Build history of the part. All positions in model axes, mm. Face numbers are marked on the shaded views. A direction names the side the tool comes from. Give positions to 0.01 mm unless a question says otherwise; leave off trailing zeros. Write each loop counter-clockwise with the first axis right and the second up, starting at its lowest first coordinate (ties: lowest second). Pieces come first, ordered by that corner, then holes.
from build123d import *

# Parameters (mm, degrees)
SKIZZE1_R                       = 125
AUFSATZ_LINEAR_AUSTRAGEN1_DEPTH = 20
SKIZZE2_R                       = 50
AUFSATZ_LINEAR_AUSTRAGEN2_DEPTH = 45
SKIZZE3_W                       = 20
SKIZZE3_H                       = 70
AUFSATZ_LINEAR_AUSTRAGEN3_DEPTH = 75
SCHNITT_LINEAR_AUSTRAGEN1_REACH = 234.403
SKIZZE5_R                       = 112.75
SKIZZE5_R_2                     = 89.75
SCHNITT_LINEAR_AUSTRAGEN2_DEPTH = 12
SKIZZE6_R                       = 15
SCHNITT_LINEAR_AUSTRAGEN3_DEPTH = 6
SKIZZE7_R                       = 6
SCHNITT_LINEAR_AUSTRAGEN4_DEPTH = 50


with BuildPart() as part:
    # Skizze1 → Aufsatz-Linear austragen1 (new body)
    with BuildSketch(Plane(origin=(0, 0, 0), x_dir=(1, 0, 0), z_dir=(0, 1, 0))):
        with Locations(Location((0, 0, 0), (0, 0, 270))):
            Circle(SKIZZE1_R)
    extrude(amount=AUFSATZ_LINEAR_AUSTRAGEN1_DEPTH)

    # Skizze2 → Aufsatz-Linear austragen2 (add)
    with BuildSketch(Plane(origin=(0, 20, 0), x_dir=(1, 0, 0), z_dir=(0, 1, 0))):
        with Locations(Location((0, 0, 0), (0, 0, 90))):
            Circle(SKIZZE2_R)
    extrude(amount=AUFSATZ_LINEAR_AUSTRAGEN2_DEPTH)

    # Skizze3 → Aufsatz-Linear austragen3 (add)
    with BuildSketch(Plane.XZ):
        with Locations((-46, 0)):
            Rectangle(SKIZZE3_W, SKIZZE3_H)
        with Locations((46, 0)):
            Rectangle(SKIZZE3_W, SKIZZE3_H)
    extrude(amount=AUFSATZ_LINEAR_AUSTRAGEN3_DEPTH)

    # Schnitt-Linear austragen1: up to this face of the body (flat: up to its plane)
    schnitt_linear_austragen1_end = Plane(part.part.faces().sort_by_distance((56, -37.5, 0))[0])
    # Skizze4 → Schnitt-Linear austragen1 (cut, up to the picked face)
    with BuildSketch(Plane.ZY.offset(56), mode=Mode.PRIVATE) as schnitt_linear_austragen1_sk1:
        with BuildLine():
            ThreePointArc((0, -75), (-24.748737342, -64.748737342), (-35, -40))
            Line((-35, -40), (-35, -75))
            Line((-35, -75), (0, -75))
        make_face()
    schnitt_linear_austragen1_tool1 = split(extrude(schnitt_linear_austragen1_sk1.sketch, amount=-SCHNITT_LINEAR_AUSTRAGEN1_REACH, mode=Mode.PRIVATE), bisect_by=schnitt_linear_austragen1_end, keep=Keep.BOTH, mode=Mode.PRIVATE)
    # Skizze4 → Schnitt-Linear austragen1 (cut, up to the picked face)
    with BuildSketch(Plane.ZY.offset(56), mode=Mode.PRIVATE) as schnitt_linear_austragen1_sk2:
        with BuildLine():
            Line((35, -75), (35, -40))
            ThreePointArc((35, -40), (24.748737342, -64.748737342), (0, -75))
            Line((0, -75), (35, -75))
        make_face()
    schnitt_linear_austragen1_tool2 = split(extrude(schnitt_linear_austragen1_sk2.sketch, amount=-SCHNITT_LINEAR_AUSTRAGEN1_REACH, mode=Mode.PRIVATE), bisect_by=schnitt_linear_austragen1_end, keep=Keep.BOTH, mode=Mode.PRIVATE)
    add(schnitt_linear_austragen1_tool1.solids().sort_by(Axis((-56, -67.182122, -27.182122), (1, 0, 0)))[0], mode=Mode.SUBTRACT)
    add(schnitt_linear_austragen1_tool2.solids().sort_by(Axis((-56, -67.182122, 27.182122), (1, 0, 0)))[0], mode=Mode.SUBTRACT)

    # Skizze5 → Schnitt-Linear austragen2 (cut)
    with BuildSketch(Plane(origin=(0, 20, 0), x_dir=(1, 0, 0), z_dir=(0, 1, 0))):
        with Locations(Location((0, 0, 0), (0, 0, 270))):
            Circle(SKIZZE5_R)
        with Locations(Location((0, 0, 0), (0, 0, 270))):
            Circle(SKIZZE5_R_2, mode=Mode.SUBTRACT)
    extrude(amount=-SCHNITT_LINEAR_AUSTRAGEN2_DEPTH, mode=Mode.SUBTRACT)

    # Skizze6 → Schnitt-Linear austragen3 (cut)
    with BuildSketch(Plane.XZ):
        with Locations(Location((0, 0, 0), (0, 0, 270))):
            Circle(SKIZZE6_R)
    extrude(amount=-SCHNITT_LINEAR_AUSTRAGEN3_DEPTH, mode=Mode.SUBTRACT)

    # Skizze7 → Schnitt-Linear austragen4 (cut)
    with BuildSketch(Plane(origin=(0, 6, 0), x_dir=(-1, 0, 0), z_dir=(0, -1, 0))):
        with Locations(Location((0, 0, 0), (0, 0, 90))):
            Circle(SKIZZE7_R)
    extrude(amount=-SCHNITT_LINEAR_AUSTRAGEN4_DEPTH, mode=Mode.SUBTRACT)


solid = part.part
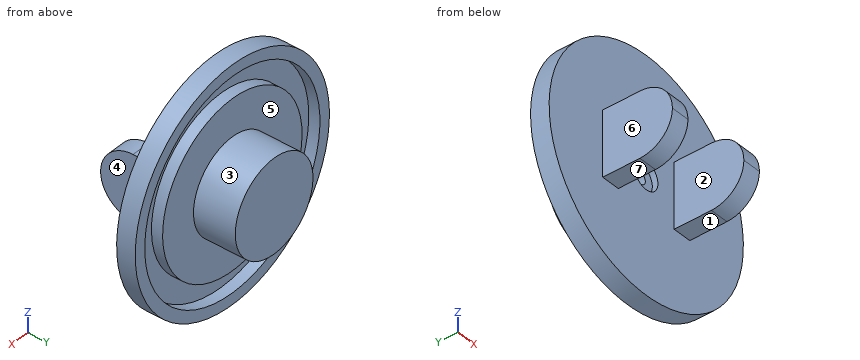
(1) Probe line 1 (X direction, y = 12.25, z = 0); line 2 (X direction, y = -19.5, z = 1.5); line 3 (X direction, y = 1.7, z = 0). List the from-to ranges inside material, lowest first.
(2) Saw through at D-D, the plane y = 37. List the corners of the cut face in (x, z).
(3) Saw through at B-B, the plane x = 0. List the corners of the cut face in (y, z).
(4) Saw through at C-C, the plane z = 31.5. List the corners of the cut face in (x, y), plus the area to 3 significant figures.
(5) Drop flat-ended pins along their axis: pin 1 (4 mm diameter, centred on x = -11, z = -88.5, fed in from +Y); pin 2 (2 mm diameter, centred on x = 25.5, z = 92.5, fed in from +Y); pin 3 (16 mm diameter, centred on x = 48.5, y = -24, fed in from +Z); pin 4 (8 mm diameter, centred on y = -41, z = 41, fed in from -X). Give the stop position or say it passes through.
(6) 3-axis set-ups, long thin cutter, end or side, ignore diameter. For the marked faces 4, 5, 6 and 7: which of +Z, -Z, +X, -X, +Y, -Y reach the whole face in a straight line?
(7) Saw through at A-A, the plane y = -18.5. List the corners of the cut face in (x, z), plus the area to 3 significant figures.
(8) Mould opens along X. For the marked faces 1, 2 and 3 say: +X half, -X half, draft (parallel to the pull), parting line (faces both ways), or undercut.
Computed values:
1. line 1: x = -125 to -112.75, -89.75 to -6, 6 to 89.75, 112.75 to 125
1. line 2: x = -56 to -36, 36 to 56
1. line 3: x = -125 to -15, 15 to 125
2. outline: circle Ø100 at (0, 0); hole circle Ø12 at (0, 0)
3. outline: (0, -125) - (20, -125) - (20, -112.75) - (8, -112.75) - (8, -89.75) - (20, -89.75) - (20, -50) - (65, -50) - (65, 50) - (20, 50) - (20, 89.75) - (8, 89.75) - (8, 112.75) - (20, 112.75) - (20, 125) - (0, 125) - (0, 15) - (6, 15) - (6, 6) - (56, 6) - (56, -6) - (6, -6) - (6, -15) - (0, -15) - close
4. outline: (-120.97, 0) - (-56, 0) - (-56, -55.26) - (-36, -55.26) - (-36, 0) - (36, 0) - (36, -55.26) - (56, -55.26) - (56, 0) - (120.97, 0) - (120.97, 20) - (108.26, 20) - (108.26, 8) - (84.04, 8) - (84.04, 20) - (38.83, 20) - (38.83, 65) - (-38.83, 65) - (-38.83, 20) - (-84.04, 20) - (-84.04, 8) - (-108.26, 8) - (-108.26, 20) - (-120.97, 20) - close
4. area: 9,960 mm2
5. pin 1: stops at y = 20
5. pin 2: stops at y = 8
5. pin 3: stops at z = 35
5. pin 4: passes through
6. face 4: +Z, -Z, +X, -Y
6. face 5: +Y
6. face 6: +Z, -Z, -X, -Y
6. face 7: -Z, +X, -X, -Y
7. outline: (-56, -35) - (-36, -35) - (-36, 35) - (-56, 35) - close; (36, -35) - (56, -35) - (56, 35) - (36, 35) - close
7. area: 2,800 mm2
8. face 1: draft
8. face 2: undercut
8. face 3: parting line
